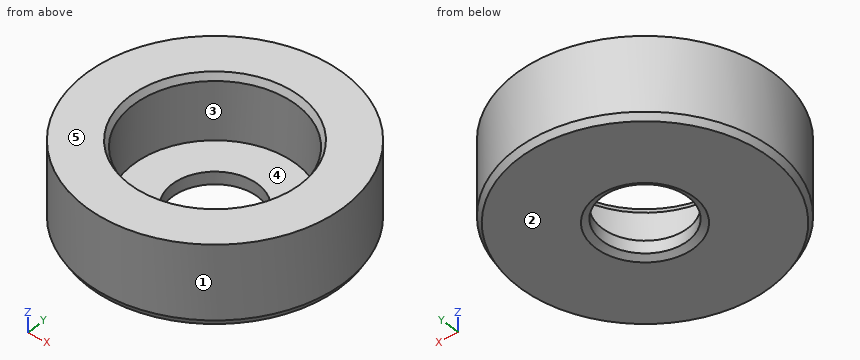
from build123d import *

# Parameters (mm, degrees)
F0_R        = 5.05
F0_R_2      = 2.65
F1_DEPTH    = 1
F0_R_3      = 8
F2_DEPTH    = 5
F3_C1_SIZE2 = 0.4
F3_C1_SIZE  = 0.2309401077
F3_C2_SIZE2 = 0.4
F3_C2_SIZE  = 0.2309401077
F3_C3_SIZE2 = 0.4
F3_C3_SIZE  = 0.2309401077


with BuildPart() as f1:
    # F0 (on Top) → F1 (new body)
    with BuildSketch(Plane.XY):
        Circle(F0_R)
        Circle(F0_R_2, mode=Mode.SUBTRACT)
    extrude(amount=F1_DEPTH)

    # F0 (on Top) → F2 (join)
    with BuildSketch(Plane.XY):
        Circle(F0_R_3)
        Circle(F0_R, mode=Mode.SUBTRACT)
    extrude(amount=F2_DEPTH)

    # F3: chamfer of 0.4 x 0.2309401077 on 3 edges, made by hand

    # F3_c1
    f3_c1_edges = [f1.edges().sort_by_distance(p)[0] for p in [
        (-2.65, 0, 0),
    ]]
    f3_c1_side = f1.faces().sort_by_distance((-2.65, 0, 0.0046188022))[0]
    chamfer(f3_c1_edges, length=F3_C1_SIZE, length2=F3_C1_SIZE2, reference=f3_c1_side)

    # F3_c2
    f3_c2_edges = [f1.edges().sort_by_distance(p)[0] for p in [
        (-8, 0, 0),
    ]]
    f3_c2_side = f1.faces().sort_by_distance((-7.9953811978, 0, 0))[0]
    chamfer(f3_c2_edges, length=F3_C2_SIZE, length2=F3_C2_SIZE2, reference=f3_c2_side)

    # F3_c3
    f3_c3_edges = [f1.edges().sort_by_distance(p)[0] for p in [
        (-5.05, 0, 5),
    ]]
    f3_c3_side = f1.faces().sort_by_distance((-5.0546188022, 0, 5))[0]
    chamfer(f3_c3_edges, length=F3_C3_SIZE, length2=F3_C3_SIZE2, reference=f3_c3_side)


solid = f1.part
Work out the finished part from the listing and answer in its coordinate system (mm). Face numbers are marked on the shaded views. A direction names the side the tool comes from. Give positions to 0.01 mm unless a question says otherwise; leave off trailing zeros. Loops run counter-clockwise (first coordinate to the right, second up) from the corner with the lowest first, then second, coordinate; pieces in that order, holes last. Notation, with made-up numbers: (21.5, 19) -> (74.5, 19) arc R27 ccw to (74.5, 58) -> close; hole circle Ø2 at (61.5, 37.5). An arc over 180 degrees is marked (long way). Use a Markdown table: item, result. Add a question column.
1. Section A-A on x = 0 is taken. Determine the outline of the cut face in (y, z).
2. Section C-C on z = 3.55 is taken. Determine the outline of the cut face in (x, y), and give its area (3 significant figures).
3. Find the intervals of material crossed by probe 1 along Y at (x, z) = (0, 0.6); probe 2 along Y at (x, z) = (0, 3.6); probe 3 along Z at (x, y) = (4.5, -1.25), in increasing order.
4. Flat-ended cylindrical pins translate along their axes: pin 1 Ø6 at (x, y) = (0, 0) entering from -Z; pin 2 Ø3 at (x, y) = (1, -1) entering from +Z; pin 3 Ø1.5 at (y, z) = (-2.5, 1) entering from +X. Find the tip coordinate at first contact, or state that the pin passes through.
5. Determine the mould class of the marked faces 1, 2 and 3 for opening direction X: released by +X, released by -X, zero draft, split by the parting line, or undercut.
6. For the marked faces 4 and 5, determine the directions among +Z, -Z, +X, -X, +Y, -Y from which every point of the face is accessible in a straight line to the end or side of a thin tool.
Results below:
| question | item | result |
|---|---|---|
| 1 | outline | (-8, 0.4) -> (-7.77, 0) -> (-3.05, 0) -> (-2.65, 0.23) -> (-2.65, 1) -> (-5.05, 1) -> (-5.05, 4.6) -> (-5.28, 5) -> (-8, 5) -> close; (2.65, 0.23) -> (3.05, 0) -> (7.77, 0) -> (8, 0.4) -> (8, 5) -> (5.28, 5) -> (5.05, 4.6) -> (5.05, 1) -> (2.65, 1) -> close |
| 2 | outline | circle Ø16 at (0, 0); hole circle Ø10.1 at (0, 0) |
| 2 | area | 121 mm^2 |
| 3 | probe 1 | y = -8 to -2.65, 2.65 to 8 |
| 3 | probe 2 | y = -8 to -5.05, 5.05 to 8 |
| 3 | probe 3 | z = 0 to 1 |
| 4 | pin 1 | stops at z = 0.03 |
| 4 | pin 2 | stops at z = 1 |
| 4 | pin 3 | stops at x = 7.81 |
| 5 | face 1 | split by the parting line |
| 5 | face 2 | zero draft |
| 5 | face 3 | undercut |
| 6 | face 4 | +Z |
| 6 | face 5 | +Z, +X, -X, +Y, -Y |
